Input: part model. Units: mm. Frame: model coordinates. Face numbers are marked on the shaded views. Round coordinates to 2 decimals unless told otherwise and drop trailing zeros. Order: outer loops, then holes, each group sorted by start corner. A loop starts at its lowest first (then second) coordinate and runs counter-clockwise, first axis right, second up.
Item 1: Cut plane A-A on z = -6.5. Output: boundary loops of the cut face in (x, y).
Item 2: Cut plane C-C on x = 73. Output: boundary loops of the cut face in (y, z), then the cut area to 3 significant figures.
Item 3: Cut plane B-B on y = 0. Output: boundary loops of the cut face in (x, z), then the cut area to 3 significant figures.
Item 4: First-contact query: pin 1 (4 mm diameter, centred on x = 142, z = -3, fed in from +Y); pin 2 (10 mm diameter, centred on x = 91.5, z = 5, fed in from +Y); pin 3 (10 mm diameter, centred on x = 75, z = 7, fed in from +Y). Flat tips, straight axial feed; report the tip coordinate or a pass-through.
Item 5: Mould query, pull axis X, two halves, no side actions, for the marked faces 1, 2 and 3. Classes: released by +X, released by -X, zero draft, split by the parting line, or undercut.
Item 6: Line query: L1, parallel to X at y = -2.5, z = -4.75; L2, parallel to Z at x = 7, y = 0; L3, parallel to X at y = -7, z = 6.25. Output: solid intervals per line, ascending.
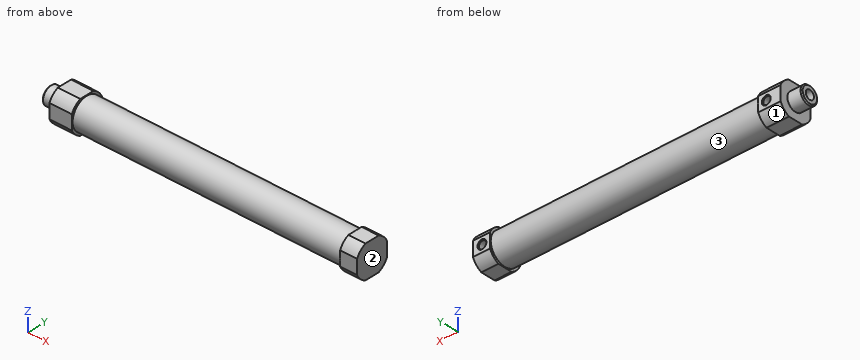
Autodesk Inventor part; units mm, degrees
ref_plane "BODY_N_XY" through (172, 0, 0) normal (0, 0, -1) x (1, 0, 0)
ref_plane "BODY_N_YZ" through (172, 0, 0) normal (1, 0, 0) x (0, -1, 0)
ref_plane "BODY_N_ZX" through (172, 0, 0) normal (0, -1, 0) x (0, 0, -1)
sketch "Sketch_8" plane through (0, 0, 0) normal (0, 0, 1) x (1, 0, 0)
  line L0 (0, 0) -> (-8, 0)
  line L1 (-8, 0) -> (-8, 4.3865)
  line L2 (-8, 4.3865) -> (-7.3865, 5)
  line L3 (-7.3865, 5) -> (0, 5)
  line L4 (0, 5) -> (0, 0)
  line L5 (0, 0) -> (-8, 0)
revolve "Revolution1" add sketch "Sketch_8" angle 360 about axis through (0, 0, 0) along (1, 0, 0)
thread "Thread1"
sketch "Sketch_9" plane through (0, 0, 0) normal (1, 0, 0) x (0, 0, -1)
  line L0 (-9.15, 4.0345) -> (-9.15, -4.0345)
  arc A0 (-9.15, -4.0345) -> (-4.0345, -9.15) centre (0, 0) ccw
  line L1 (-4.0345, -9.15) -> (4.0345, -9.15)
  arc A1 (4.0345, -9.15) -> (9.15, -4.0345) centre (0, 0) ccw
  line L2 (9.15, -4.0345) -> (9.15, 4.0345)
  arc A2 (9.15, 4.0345) -> (4.0345, 9.15) centre (0, 0) ccw
  line L3 (4.0345, 9.15) -> (-4.0345, 9.15)
  arc A3 (-4.0345, 9.15) -> (-9.15, 4.0345) centre (0, 0) ccw
extrude "Extrusion1" add sketch "Sketch_9" along normal blind 12.5
sketch "Sketch_11" plane through (12.5, 0, 0) normal (1, 0, 0) x (0, 0, -1)
  circle A0 centre (0, 0) radius 8.7
extrude "Extrusion2" add sketch "Sketch_11" along normal blind 150
sketch "Sketch_10" plane through (162.5, 0, 0) normal (1, 0, 0) x (0, 0, -1)
  line L0 (-9.15, 4.0345) -> (-9.15, -4.0345)
  arc A0 (-9.15, -4.0345) -> (-4.0345, -9.15) centre (0, 0) ccw
  line L1 (-4.0345, -9.15) -> (4.0345, -9.15)
  arc A1 (4.0345, -9.15) -> (9.15, -4.0345) centre (0, 0) ccw
  line L2 (9.15, -4.0345) -> (9.15, 4.0345)
  arc A2 (9.15, 4.0345) -> (4.0345, 9.15) centre (0, 0) ccw
  line L3 (4.0345, 9.15) -> (-4.0345, 9.15)
  arc A3 (-4.0345, 9.15) -> (-9.15, 4.0345) centre (0, 0) ccw
extrude "Extrusion3" add sketch "Sketch_10" along normal blind 9.5
sketch "Sketch7" plane through (0, 0, 0) normal (0, 0, 1) x (1, 0, 0)
  line L0 (8, 9.15) -> (8, 4.15)
  line L1 (8, 2.9566) -> (5.933, 4.15)
  line L2 (5.933, 4.15) -> (5.933, 8.717)
  line L3 (5.933, 8.717) -> (5.5, 9.15)
  line L4 (5.5, 9.15) -> (8, 9.15)
  line L5 (8, 9.15) -> (8, 2.9566)
revolve "Revolution2" cut sketch "Sketch7" angle 360 about axis through (8, 9.15, 0) along (0, 1, 0)
thread "Thread2"
sketch "Sketch_7" plane through (0, 0, 0) normal (0, 0, 1) x (1, 0, 0)
  line L0 (167, 9.15) -> (167, 4.15)
  line L1 (167, 2.9566) -> (164.933, 4.15)
  line L2 (164.933, 4.15) -> (164.933, 8.717)
  line L3 (164.933, 8.717) -> (164.5, 9.15)
  line L4 (164.5, 9.15) -> (167, 9.15)
  line L5 (167, 9.15) -> (167, 2.9566)
revolve "Revolution3" cut sketch "Sketch_7" angle 360 about axis through (167, 9.15, 0) along (0, 1, 0)
thread "Thread3"
sketch "Sketch_16" plane through (0, 0, 0) normal (0, 0, 1) x (1, 0, 0)
  line L0 (142.5, 0) -> (-8, 0)
  line L1 (-8, 0) -> (-8, 2.5)
  line L2 (-8, 2.5) -> (12.5, 2.5)
  line L3 (12.5, 2.5) -> (12.5, 8)
  line L4 (12.5, 8) -> (142.5, 8)
  line L5 (142.5, 8) -> (142.5, 0)
  line L6 (142.5, 0) -> (-8, 0)
revolve "Revolution4" cut sketch "Sketch_16" angle 360 about axis through (142.5, 0, 0) along (1, 0, 0)
ref_plane "BODY_N_XY" through (172, 0, 0) normal (0, 0, -1) x (1, 0, 0)
ref_plane "BODY_N_YZ" through (172, 0, 0) normal (1, 0, 0) x (0, -1, 0)
ref_plane "BODY_N_ZX" through (172, 0, 0) normal (0, -1, 0) x (0, 0, -1)
ref_plane "NUT2_XY" through (172, 0, 0) normal (1, 0, 0) x (0, 0, -1)
ref_plane "NUT2_YZ" through (172, 0, 0) normal (0, 0, -1) x (0, 1, 0)
ref_plane "NUT2_ZX" through (172, 0, 0) normal (0, 1, 0) x (1, 0, 0)
ref_plane "SW1_XY" through (17.5, 0, 0) normal (1, 0, 0) x (0, 0, -1)
ref_plane "SW1_YZ" through (17.5, 0, 0) normal (0, 0, -1) x (0, 1, 0)
ref_plane "SW1_ZX" through (17.5, 0, 0) normal (0, 1, 0) x (1, 0, 0)
ref_plane "SW2_XY" through (157.5, 0, 0) normal (-1, 0, 0) x (0, 0, -1)
ref_plane "SW2_YZ" through (157.5, 0, 0) normal (0, 0, -1) x (0, -1, 0)
ref_plane "SW2_ZX" through (157.5, 0, 0) normal (0, -1, 0) x (-1, 0, 0)
ref_plane "SW_R1_XY" through (17.5, -14.15, 0) normal (1, 0, 0) x (0, 0, -1)
ref_plane "SW_R1_YZ" through (17.5, -14.15, 0) normal (0, 0, -1) x (0, 1, 0)
ref_plane "SW_R1_ZX" through (17.5, -14.15, 0) normal (0, 1, 0) x (1, 0, 0)
ref_plane "SW_R2_XY" through (157.5, -14.15, 0) normal (-1, 0, 0) x (0, 0, -1)
ref_plane "SW_R2_YZ" through (157.5, -14.15, 0) normal (0, 0, -1) x (0, -1, 0)
ref_plane "SW_R2_ZX" through (157.5, -14.15, 0) normal (0, -1, 0) x (-1, 0, 0)
ref_plane "body_XY" through (0, 0, 0) normal (1, 0, 0) x (0, 0, -1)
ref_plane "body_YZ" through (0, 0, 0) normal (0, 0, -1) x (0, 1, 0)
ref_plane "body_ZX" through (0, 0, 0) normal (0, 1, 0) x (1, 0, 0)
properties part number "CJ2B16-125Z(1_0)_BODY" material "ステンレス鋼"
From the geometry:
1. outline: (0, -7.6) - (12.5, -7.6) - (12.5, -5.78) - (162.5, -5.78) - (162.5, -7.6) - (172, -7.6) - (172, 7.6) - (162.5, 7.6) - (162.5, 5.78) - (12.5, 5.78) - (12.5, 7.6) - (0, 7.6) - close; hole (12.5, -4.66) - (142.5, -4.66) - (142.5, 4.66) - (12.5, 4.66) - close
2. outline: circle Ø17.4 at (0, 0); hole circle Ø16 at (0, 0)
2. area: 36.7 mm2
3. outline: (-8, -4.39) - (-7.39, -5) - (0, -5) - (0, -9.15) - (12.5, -9.15) - (12.5, -8.7) - (162.5, -8.7) - (162.5, -9.15) - (172, -9.15) - (172, 9.15) - (162.5, 9.15) - (162.5, 8.7) - (12.5, 8.7) - (12.5, 9.15) - (0, 9.15) - (0, 5) - (-7.39, 5) - (-8, 4.39) - (-8, 2.5) - (12.5, 2.5) - (12.5, 8) - (142.5, 8) - (142.5, -8) - (12.5, -8) - (12.5, -2.5) - (-8, -2.5) - close
3. area: 910 mm2
4. pin 1: stops at y = 8.64
4. pin 2: stops at y = 8.7
4. pin 3: stops at y = 8.47
5. face 1: zero draft
5. face 2: released by +X
5. face 3: undercut
6. L1: x = 0 to 12.5, 142.5 to 172
6. L2: z = -9.15 to -2.5, 2.5 to 9.15
6. L3: x = 0 to 12.5, 162.5 to 172
